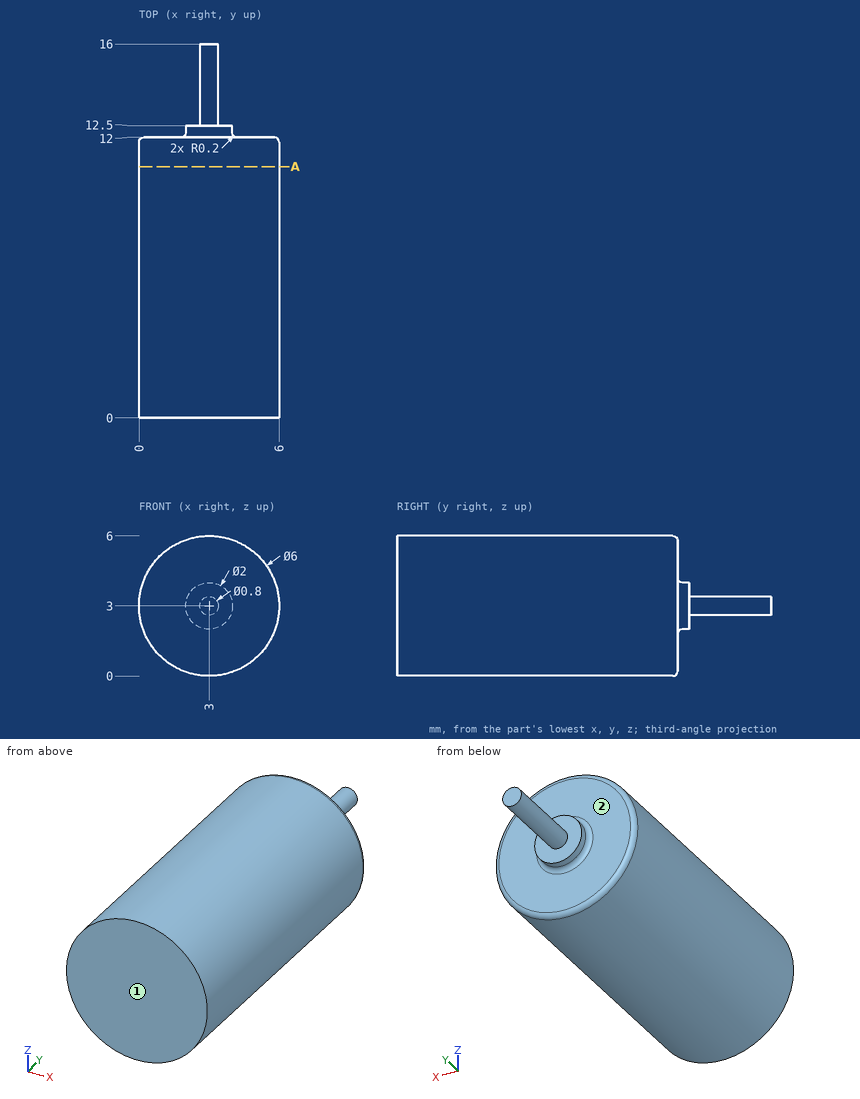
Verification items for this drawing (mm, ordinates from the low corner). A direction names the side the tool comes from. Round coordinates to 2 decimals unless told otherwise and drop trailing zeros. Order: outer loops, then holes, each group sorted by start corner. A loop starts at its lowest first (then second) coordinate and runs counter-clockwise, first axis right, second up. Notation, with made-up numbers: (54.25, 51.5) - (62.25, 51.5) arc R33 ccw to (62.25, 83.5) - close; hole circle Ø1 at (40, 71.5). An arc over 180 degrees is marked (long way). Use CSV: the item, a comma, the result in double quotes.
(1) Section check A-A on y = 10.75. Record the boundary of the cut face in (x, z).
Entries:
outline,"circle Ø6 at (3, 3)"
(2) Gauge pin test, flat end, axial feed: pin 1 Ø3 at (x, y) = (1, 13) entering from -Z. Record the tip position at first contact, or that the pin passes through.
Entries:
pin 1,"z = 0.19"
(3) Thickness scan on probe 1 along Y at (x, z) = (1.5, 4.5); probe 2 along Z at (x, y) = (0.25, 7.5); probe 3 along Y at (x, z) = (3.75, 3.25). Record the ranges inside material, lowest first. Write a range as from..to.
Entries:
probe 1,"0..12"
probe 2,"1.8..4.2"
probe 3,"0..12.5"
(4) Access from +Z, -Z, +X, -X, +Y, -Y to the whole of each face (thin tool, end or side, straight path). Record for the marked faces 1 and 2.
Entries:
face 1,"+Z, -Z, +X, -X, -Y"
face 2,"+Y"
